Check sheet for the drawn part. Datum: minimum x, y, z corner. Units: mm. A direction names the side the tool comes from. Round coordinates to 2 decimals unless told otherwise and drop trailing zeros. Loops run counter-clockwise (first coordinate to the right, second up) from the corner with the lowest first, then second, coordinate; pieces in that order, holes last.
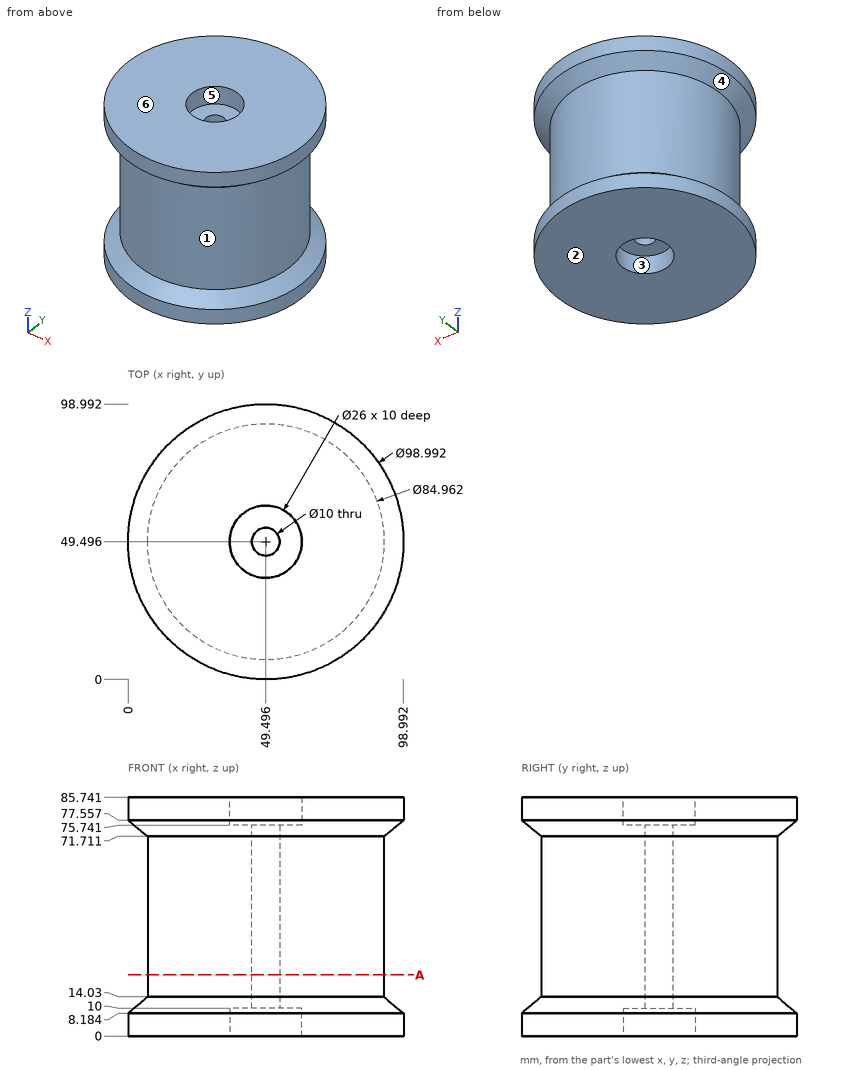
1) Mould release check, pull along Y, two halves, no side actions. Record for the marked faces 4, 5 and 6: +Y half, -Y half, draft (parallel to the pull), parting line (faces both ways), or undercut.
Report:
face 4: parting line
face 5: undercut
face 6: draft
2) Gauge pin test, flat ends, axial feed: pin 1 (5 mm diameter, centred on y = 69, z = 66, fed in from +X) (1 decimal); pin 2 (12 mm diameter, centred on x = 60.5, z = 68.5, fed in from +Y) (1 decimal); pin 3 (5 mm diameter, centred on y = 79.5, z = 65, fed in from -X). Record the tip position at first contact, or that the pin passes through.
Report:
pin 1: stops at x = 88.4
pin 2: stops at y = 94.1
pin 3: stops at x = 17.12
3) Sectioned sample at A-A, the plane z = 22. Record the cut outline in (x, y) (1 decimal).
Report:
outline: circle Ø85 at (49.5, 49.5); hole circle Ø10 at (49.5, 49.5)
4) Scan lines: line 1 along X through (y, z) = (48.5, 58) (1 decimal); line 2 along Z through (x, y) = (28.5, 93.5); line 3 along Y through (x, z) = (45.5, 37.5) (1 decimal). Record each from-to range of solid material in increasing order.
Report:
line 1: x = 7 to 44.6, 54.4 to 92
line 2: z = 0 to 8.8, 76.94 to 85.74
line 3: y = 7.2 to 46.5, 52.5 to 91.8
5) Access from +Z, -Z, +X, -X, +Y, -Y to the whole of each face (thin tool, end or side, straight path). Record for the marked faces 1, 2 and 3.
Report:
face 1: none
face 2: -Z, +X, -X, +Y, -Y
face 3: -Z
